For this review, take the finished solid that the model builds, in its own axes (mm). A direction names the side the tool comes from. Give positions to 0.01 mm unless a question says otherwise; leave off trailing zeros. Loops run counter-clockwise (first coordinate to the right, second up) from the corner with the lowest first, then second, coordinate; pieces in that order, holes last. Notation, with made-up numbers: (13, -4) - (39, -4) arc R23 ccw to (39, 10) - close; hole circle Ø10 at (35.5, 77). An arc over 180 degrees is marked (long way). Answer in a Markdown table with one row per item.
```python
from build123d import *

# Parameters (mm, degrees)
SKETCH1_W              = 165.1
SKETCH1_H              = 165.1
SKETCH1_W_2            = 139.7
SKETCH1_H_2            = 139.7
BOSS_EXTRUDE1_DEPTH    = 6.35
FILLET1_R              = 6.35
F_10_32_TAPPED_HOLE1_D = 4.0386
SKETCH4_OUTSIDE_W      = 213.814
SKETCH4_OUTSIDE_H      = 213.814
SKETCH4_OUTSIDE_R      = 6.35
CUT_EXTRUDE1_DEPTH     = 3.175


with BuildPart() as part:
    # Sketch1 → Boss-Extrude1 (new body)
    with BuildSketch(Plane(origin=(0, 0, 0), x_dir=(1, 0, 0), z_dir=(0, 1, 0))):
        Rectangle(SKETCH1_W, SKETCH1_H)
        Rectangle(SKETCH1_W_2, SKETCH1_H_2, mode=Mode.SUBTRACT)
    extrude(amount=BOSS_EXTRUDE1_DEPTH)

    # Fillet1
    fillet1_edges = [part.edges().sort_by_distance(p)[0] for p in [
        (-69.85, 3.175, -69.85),
        (-69.85, 3.175, 69.85),
        (69.85, 3.175, 69.85),
        (69.85, 3.175, -69.85),
        (-82.55, 3.175, -82.55),
        (82.55, 3.175, -82.55),
        (82.55, 3.175, 82.55),
        (-82.55, 3.175, 82.55),
    ]]
    fillet(fillet1_edges, radius=FILLET1_R)

    # #10-32 Tapped Hole1 (through all)
    with Locations(Plane(origin=(0, 6.35, 0), x_dir=(1, 0, 0), z_dir=(0, 1, 0))):
        with Locations((-76.2, -76.2), (-76.2, 76.2), (76.2, 76.2), (76.2, -76.2), (-76.2, 0), (0, 76.2), (76.2, 0), (0, -76.2)):
            Hole(F_10_32_TAPPED_HOLE1_D / 2)

    # Sketch4 outside → Cut-Extrude1 (cut)
    with BuildSketch(Plane(origin=(0, 6.35, 0), x_dir=(1, 0, 0), z_dir=(0, 1, 0))):
        Rectangle(SKETCH4_OUTSIDE_W, SKETCH4_OUTSIDE_H)
        with Locations(Location((-76.2, 76.2, 0), (0, 0, 90))):
            Circle(SKETCH4_OUTSIDE_R, mode=Mode.SUBTRACT)
        with Locations(Location((-76.2, 0, 0), (0, 0, 270))):
            Circle(SKETCH4_OUTSIDE_R, mode=Mode.SUBTRACT)
        with Locations(Location((-76.2, -76.2, 0), (0, 0, 270))):
            Circle(SKETCH4_OUTSIDE_R, mode=Mode.SUBTRACT)
        with Locations(Location((0, -76.2, 0), (0, 0, 270))):
            Circle(SKETCH4_OUTSIDE_R, mode=Mode.SUBTRACT)
        with Locations(Location((76.2, -76.2, 0), (0, 0, 270))):
            Circle(SKETCH4_OUTSIDE_R, mode=Mode.SUBTRACT)
        with Locations(Location((76.2, 0, 0), (0, 0, 270))):
            Circle(SKETCH4_OUTSIDE_R, mode=Mode.SUBTRACT)
        with Locations(Location((76.2, 76.2, 0), (0, 0, 90))):
            Circle(SKETCH4_OUTSIDE_R, mode=Mode.SUBTRACT)
        with Locations(Location((0, 76.2, 0), (0, 0, 270))):
            Circle(SKETCH4_OUTSIDE_R, mode=Mode.SUBTRACT)
    extrude(amount=-CUT_EXTRUDE1_DEPTH, mode=Mode.SUBTRACT)


solid = part.part
```
1. For faces 3 (the face through (-67.94, 1.61, -68.04)), 4 (the face through (-57, 3.175, 72)), 5 (the face through (76, 6.35, -73)), list the 3-axis set-ups (+Z, -Z, +X, -X, +Y, -Y) from which the entire face can be reached by the end or side of a thin tool; tool diameter is ignored.
Values:
| item | result |
|---|---|
| face 3 | +Y, -Y |
| face 4 | +Y |
| face 5 | +Z, -Z, +X, -X, +Y |
2. We need section B-B, the plane z = -35. Give the boundary of the cut face in (x, y) (3 decimals).
Values:
| item | result |
|---|---|
| outline | (-82.55, 0) - (-69.85, 0) - (-69.85, 3.175) - (-82.55, 3.175) - close; (69.85, 0) - (82.55, 0) - (82.55, 3.175) - (69.85, 3.175) - close |
3. We need section C-C, the plane x = 54.5. Give the boundary of the cut face in (y, z) (3 decimals).
Values:
| item | result |
|---|---|
| outline | (0, -82.55) - (3.175, -82.55) - (3.175, -69.85) - (0, -69.85) - close; (0, 69.85) - (3.175, 69.85) - (3.175, 82.55) - (0, 82.55) - close |
4. We need section A-A, the plane y = 5. Count the separate pieces of the cut face and the enclosed holes in it, and give its area (3 significant figures).
Values:
| item | result |
|---|---|
| separate pieces | 8 |
| enclosed holes | 8 |
| area | 911 mm^2 |
5. Wall thickness on line 1 (Z direction, x = -76.2, y = 2.5); line 2 (Z direction, x = 0, y = 2.75); line 3 (X direction, y = 5.25, z = -76.2): over which ranges is each line inside the solid? List them lowest first. Write a range as [from, to].
Values:
| item | result |
|---|---|
| line 1 | z = [-82.55, -78.22], [-74.18, -2.02], [2.02, 74.18], [78.22, 82.55] |
| line 2 | z = [-82.55, -78.22], [-74.18, -69.85], [69.85, 74.18], [78.22, 82.55] |
| line 3 | x = [-82.55, -78.22], [-74.18, -69.85], [-6.35, -2.02], [2.02, 6.35], [69.85, 74.18], [78.22, 82.55] |
6. Mouldability with a two-part tool opening along X and no side actions: class faces 1 (the face through (-78, 6.35, -78)), 2 (the face through (78.107, 3.925, 82.257)) as released by +X, released by -X, zero draft, split by the parting line, or undercut.
Values:
| item | result |
|---|---|
| face 1 | zero draft |
| face 2 | undercut |
